Model file for the job. Use its own axes, mm. A direction names the side the tool comes from. Coordinates: 2 decimals unless noted, no trailing zeros. Order: outer loops, then holes, each group sorted by start corner. A loop starts at its lowest first (then second) coordinate and runs counter-clockwise, first axis right, second up. Notation, with made-up numbers: M 81,51 L 119,51 A10 ccw 119,67 Z; hole C 52.5,4.5 d1. An arc over 180 degrees is marked long. Return JSON: item names as keys, results as strings.
Autodesk Inventor part; units mm, degrees
ref_plane "YZ Plane" through (0, 0, 0) normal (1, 0, 0) x (0, 1, 0)
ref_plane "XZ Plane" through (0, 0, 0) normal (0, 1, 0) x (-1, 0, 0)
ref_plane "XY Plane" through (0, 0, 0) normal (0, 0, 1) x (1, 0, 0)
sketch "Sketch1" plane through (0, 0, 0) normal (0, 1, 0) x (-1, 0, 0)
  line L0 (15, -7.5) -> (-15, -7.5)
  line L1 (-15, -7.5) -> (-15, 7.5)
  line L2 (-15, 7.5) -> (15, 7.5)
  line L3 (15, 7.5) -> (15, -7.5)
  line L4 (15, -7.5) -> (-15, 7.5) construction
  line L5 (-15, -7.5) -> (15, 7.5) construction
  point P0 (0, 0)
  dimension "d10" = 30
  dimension "d11" = 15
extrude "Plate1" add sketch "Sketch1" along normal blind 1.5875
sketch "Sketch3" plane through (15, 0, 7.5) normal (1, 0, 0) x (0, 0, -1)
  line L0 (15, 0) -> (15, 1.5875)
  line L1 (15, 0) -> (15, 46.5147)
  line L2 (15, 0) -> (0, 0)
  line L3 (15, 63.4853) -> (15, 75)
  line L4 (6.5147, 55) -> (15, 46.5147)
  line L5 (15, 63.4853) -> (6.5147, 55)
  point P0 (7.5, 0)
  point P1 (15, 55)
  dimension "d48" = 75
  dimension "d91" = 55
  dimension "d92" = 0
  dimension "d94" = 90
  dimension "d95" = 135
  dimension "d96" = 6
  dimension "d97" = 6
contour flange "Contour Flange4" sketch "Sketch3" thickness 1.5875 bend radius 1.5875 curves L1 L4 L5 L3 edges at (0, 1.5875, -7.5) running between points at (15, 1.5875, -7.5) (-15, 1.5875, -7.5)
bend "Bend4"
corner "Corner4"
sketch "Sketch4" plane through (-15, 75, -5.9125) normal (0, 0, 1) x (1, 0, 0)
  line L0 (0, -10.1996) -> (30, -10.1996)
  line L1 (30, 0) -> (0, 0)
  line L2 (0, 0) -> (0, -10.1996)
  circle A0 centre (7.5, -5) radius 1.5
  line L3 (15, 0) -> (15, -10.1996)
  circle A1 centre (22.5, -5) radius 1.5
  point P0 (15, -75)
  dimension "d50" = 3
  dimension "d52" = 5
  dimension "d53" = 7.5
extrude "Cut1" cut sketch "Sketch4" against normal blind 1.5875 contours A0 | A1
sketch "Sketch9" plane through (-15, 45.1996, -5.9125) normal (0, 0, 1) x (1, 0, 0)
  line L0 (0, 0) -> (30, 0)
  line L1 (0, 0) -> (0, -42.0246)
  line L2 (0, -42.0246) -> (30, -42.0246)
  line L3 (30, 0) -> (30, -42.0246)
  circle A0 centre (7.5, -5.1996) radius 1.5
  line L4 (15, -42.0246) -> (15, 0)
  line L5 (0, -5.1996) -> (30, -5.1996)
  circle A1 centre (22.5, -5.1996) radius 1.5
  circle A2 centre (22.5, 24.8004) radius 1.5
  point P0 (15, -45.1996)
  dimension "d79" = 3
  dimension "d81" = 7.5
  dimension "d84" = 30
extrude "Cut4" cut sketch "Sketch9" against normal blind 1.5875 contours L5 A0 | A0 L5 | A1 L5 | L5 A1
sketch "Sketch8" plane through (0, 0, 0) normal (0, -1, 0) x (1, 0, 0)
  line L0 (0, 0) -> (-15, 0)
  line L1 (-15, 0) -> (-15, 7.5)
  line L2 (-15, 7.5) -> (0, 7.5)
  line L3 (0, 7.5) -> (0, 0)
  circle A0 centre (-10, 0) radius 1.5
  circle A1 centre (10, 0) radius 1.5
  dimension "d75" = 3
  dimension "d76" = 5
extrude "Cut3" cut sketch "Sketch8" against normal blind 1.5875 contours A0 L0 | L0 A0 | A1
equation "\"d10\" = laser_x"
equation "\"d11\" = laser_y"
equation "\"d48\" = laser_z"
equation "\"d50\" = m3_diameter"
equation "\"d53\" = 0.25 * laser_x"
equation "\"d54\" = Thickness"
equation "\"d79\" = m3_diameter"
equation "\"d81\" = 0.25 * laser_x"
equation "\"d82\" = Thickness"
equation "\"d75\" = m3_diameter"
equation "\"d76\" = 0.166667 * laser_x"
equation "\"d77\" = Thickness"
equation "\"Thickness\" = sm_thickness"
equation "\"d36\" = BendReliefWidth"
equation "\"d37\" = BendReliefDepth"
equation "\"d38\" = MinimumRemnant"
equation "\"d39\" = BendRadius"
equation "\"d40\" = BendRadius"
equation "\"d42\" = CornerReliefSize"
equation "\"d43\" = GapSize"
equation "\"d44\" = JacobiRadiusSize"
equation "\"BendRadius\" = Thickness"
equation "\"BendReliefWidth\" = Thickness"
equation "\"BendReliefDepth\" = 0.5 * Thickness"
equation "\"CornerReliefSize\" = 4 * Thickness"
equation "\"MinimumRemnant\" = 2 * Thickness"
equation "\"TransitionRadius\" = BendRadius"
equation "\"JacobiRadiusSize\" = BendRadius"
equation "\"GapSize\" = Thickness"
equation "\"d0\" = BendRadius"
equation "\"sm_thickness\" = 1.5875"
equation "\"very_thick_acrylic\" = 9.45"
equation "\"thick_acrylic\" = 5.88"
equation "\"thin_acrylic\" = 3.15"
equation "\"clear_acrylic\" = 3.15"
equation "\"wood_thickness\" = 6.72"
equation "\"m3_diameter\" = 3"
equation "\"m3_head\" = 6"
equation "\"m4_diameter\" = 4"
equation "\"m5_diameter\" = 5"
equation "\"m5_head\" = 10.3"
equation "\"brass_insert_drill\" = 4"
equation "\"m5_brass_insert_drill\" = 6.7"
equation "\"m3_press_nut_drill\" = 4.5"
equation "\"m5_press_nut_drill\" = 6.5"
equation "\"stepper_screw_space\" = 35"
equation "\"stepper_shaft_diameter\" = 5"
equation "\"stepper_body_diameter\" = 28"
equation "\"laser_body_diameter\" = 12"
equation "\"carrier_y\" = 251"
equation "\"carrier_z\" = 12"
equation "\"visor_x\" = 253.925"
equation "\"visor_y\" = 85.6"
equation "\"window_z\" = 332.225"
equation "\"window_y\" = 93.75"
equation "\"window_overlap\" = 48"
equation "\"acrylic_into_frame\" = 5"
equation "\"door_x\" = 251"
equation "\"door_z\" = 332.225"
equation "\"door_overlap\" = 48"
equation "\"reservoir_x\" = 201"
equation "\"reservoir_y\" = 201"
equation "\"linear_bearing_spacing\" = 271"
equation "\"tray_border\" = 25"
equation "\"tray_x\" = 251"
equation "\"tray_y\" = 251"
equation "\"bed_z\" = 25"
equation "\"crane_z2\" = 12"
equation "\"end_stop_spacing\" = 19"
equation "\"thumb_nut_offset_y\" = 0"
equation "\"thumb_nut_diameter\" = 7"
equation "\"z_min_from_center\" = 115"
equation "\"frame_top_z\" = 385"
equation "\"frame_bottom_z\" = 275"
equation "\"frame_total_z\" = 661.5875"
equation "\"frame_border\" = 48.0375"
equation "\"frame_foot_z\" = 12"
equation "\"frame_tilt\" = 1deg"
equation "\"subframe_x\" = 66"
equation "\"subframe_y_offset\" = 27.5"
equation "\"laser_y_offset\" = 19.4"
equation "\"laser_diameter\" = 12"
equation "\"laser_z_offset\" = 55"
equation "\"laser_y\" = 15"
equation "\"laser_z\" = 75"
equation "\"laser_x\" = 30"
equation "\"t_galvo_frame\" = 6.72"
equation "\"galvo_frame_x\" = 66"
equation "\"galvo_frame_z\" = 85"
equation "\"galvo_frame_y_offset\" = 27.5"
equation "\"drawer_x\" = 257.3"
equation "\"drawer_y\" = 90.3375"
equation "\"drawer_z\" = 278.175"
equation "\"drawer_support_from_top\" = 48"
equation "\"nema17_x\" = 43"
equation "\"laser_gap\" = 1"
equation "\"frame_screw_from_center\" = 25"
equation "\"drawer_screw_from_center\" = 55"
equation "\"frame_face_y\" = 45"
equation "\"switch_spacing\" = 19"
equation "\"subframe_y\" = 55"
equation "\"al_thickness\" = 1.5875"
equation "\"rivet_diameter\" = 3.3"
equation "\"bend_factor\" = 2.26205"
equation "\"al_bend\" = 3.591"
equation "\"sm_bend\" = 3.591"
equation "\"frame_x\" = 353.375"
equation "\"carrier_z2\" = 25"
equation "\"carrier_y2\" = 76.825"
properties part number "laserholder"
Item 1: Wall check: line 1 (X direction, y = 40, z = -6.2); line 2 (Y direction, x = -4.5, z = -4.25); line 3 (Y direction, x = 7.25, z = -2.75). Give the ranges that are in metal, low to high.
Check result:
{"line 1": "x = -15 to -9, -6 to 6, 9 to 15", "line 2": "y = 0 to 1.59, 47.52 to 49.76, 60.24 to 62.48", "line 3": "y = 0 to 1.59, 49.02 to 51.26, 58.74 to 60.98"}
Item 2: Pull direction Z, two halves, no side cores. Call faces 4 (the flat face through (15, 29.3, -6.1)), 5 (the cylindrical face through (8.5, 0.78, 0.07)), 6 (the flat face through (-0.21, 59.384, -3.399)): +Z half, -Z half, draft (parallel to the pull), parting line (faces both ways), or undercut.
Check result:
{"face 4": "draft", "face 5": "undercut", "face 6": "-Z half"}
Item 3: Drop flat-ended pins along their axis: pin 1 Ø4 at (x, z) = (10, 0) entering from +Y; pin 2 Ø5 at (x, y) = (-7.5, 70) entering from +Z; pin 3 Ø8 at (x, y) = (-2, 59) entering from -Z. Give the stop position or say it passes through.
Check result:
{"pin 1": "stops at y = 60.23", "pin 2": "stops at z = -5.91", "pin 3": "stops at z = -6.94"}
Item 4: 3-axis set-ups, long thin cutter, end or side, ignore diameter. For faces 1 (the flat face through (0, 70, -5.912)), 2 (the cylindrical face through (-0.21, 2.065, -5.46)), 3 (the flat face through (-0.21, 50.706, -3.309)): which of +Z, -Z, +X, -X, +Y, -Y reach the whole face in a straight line?
Check result:
{"face 1": "+Z, +X, -X, +Y", "face 2": "+Z, +X, -X", "face 3": "-Z, +X, -X"}
Item 5: Saw through at D-D (z = 5). Write the cut outline in (x, y).
Check result:
{"outline": "M -15,0 L 15,0 L 15,1.59 L -15,1.59 Z"}
Item 6: Saw through at B-B (y = 70). Write the cut outline in (x, z), and give its area (3 significant figures).
Check result:
{"outline": "M -15,-7.5 L -9,-7.5 L -9,-5.91 L -15,-5.91 Z; M -6,-7.5 L 6,-7.5 L 6,-5.91 L -6,-5.91 Z; M 9,-7.5 L 15,-7.5 L 15,-5.91 L 9,-5.91 Z", "area": "38.1 mm2"}
